```python
from build123d import *

# Parameters (mm, degrees)
F0_W     = 600
F0_H     = 600
F0_R     = 19
F1_DEPTH = 10


with BuildPart() as f1:
    # F0 (on Top) → F1 (new body)
    with BuildSketch(Plane.XY):
        with Locations((24.970765, 120.387087)):
            Rectangle(F0_W, F0_H)
        with Locations((-220.029235, -124.612913)):
            Circle(F0_R, mode=Mode.SUBTRACT)
        with Locations((-100.029235, -124.612913)):
            Circle(F0_R, mode=Mode.SUBTRACT)
        with Locations((19.970765, -124.612913)):
            Circle(F0_R, mode=Mode.SUBTRACT)
        with Locations((-220.029235, -4.612913)):
            Circle(F0_R, mode=Mode.SUBTRACT)
        with Locations((-220.029235, 115.387087)):
            Circle(F0_R, mode=Mode.SUBTRACT)
        with Locations((-100.029235, -4.612913)):
            Circle(F0_R, mode=Mode.SUBTRACT)
        with Locations((19.970765, -4.612913)):
            Circle(F0_R, mode=Mode.SUBTRACT)
        with Locations((-100.029235, 115.387087)):
            Circle(F0_R, mode=Mode.SUBTRACT)
        with Locations((19.970765, 115.387087)):
            Circle(F0_R, mode=Mode.SUBTRACT)
        with Locations((139.970765, -124.612913)):
            Circle(F0_R, mode=Mode.SUBTRACT)
        with Locations((259.970765, -124.612913)):
            Circle(F0_R, mode=Mode.SUBTRACT)
        with Locations((139.970765, -4.612913)):
            Circle(F0_R, mode=Mode.SUBTRACT)
        with Locations((139.970765, 115.387087)):
            Circle(F0_R, mode=Mode.SUBTRACT)
        with Locations((259.970765, -4.612913)):
            Circle(F0_R, mode=Mode.SUBTRACT)
        with Locations((259.970765, 115.387087)):
            Circle(F0_R, mode=Mode.SUBTRACT)
        with Locations((-220.029235, 235.387087)):
            Circle(F0_R, mode=Mode.SUBTRACT)
        with Locations((-100.029235, 235.387087)):
            Circle(F0_R, mode=Mode.SUBTRACT)
        with Locations((19.970765, 235.387087)):
            Circle(F0_R, mode=Mode.SUBTRACT)
        with Locations((-220.029235, 355.387087)):
            Circle(F0_R, mode=Mode.SUBTRACT)
        with Locations((-100.029235, 355.387087)):
            Circle(F0_R, mode=Mode.SUBTRACT)
        with Locations((19.970765, 355.387087)):
            Circle(F0_R, mode=Mode.SUBTRACT)
        with Locations((139.970765, 235.387087)):
            Circle(F0_R, mode=Mode.SUBTRACT)
        with Locations((259.970765, 235.387087)):
            Circle(F0_R, mode=Mode.SUBTRACT)
        with Locations((139.970765, 355.387087)):
            Circle(F0_R, mode=Mode.SUBTRACT)
        with Locations((259.970765, 355.387087)):
            Circle(F0_R, mode=Mode.SUBTRACT)
    extrude(amount=-F1_DEPTH)


solid = f1.part
```
Can you work these out from the model? Positions are in its coordinate system, mm. Round coordinates to 2 decimals unless told otherwise and drop trailing zeros. Order: outer loops, then holes, each group sorted by start corner. A loop starts at its lowest first (then second) coordinate and runs counter-clockwise, first axis right, second up. Notation, with made-up numbers: (63, 8.25) -> (84, 8.25) arc R9 cw to (84, 13.25) -> close; hole circle Ø10 at (55, 7). An arc over 180 degrees is marked (long way). Return JSON: item names as keys, results as strings. Group by question number.
1. If we section it at A-A, the plane y = -15.5: Write out the boundary of the cut face in (x, z).
2. If we section it at B-B, the plane z = -5.75: Count the separate pieces of the cut face and the enclosed holes in it, then the cut area to 3 significant figures.
3. Will this pin go through, and if not, where does the flat tip stop? pin 1 (23 mm diameter, centred on x = -220.03, y = -4.61, fed in from +Z).
4. I need wall thicknesses on line 1 (Y direction, x = -223, z = -6.5); line 2 (Y direction, x = 245, z = -7.75); line 3 (X direction, y = 131.5, z = -5.75). Which ranges of each line are inside material? Lowest first, please. Write a range as [from, to].
5. We'd pull the mould along Y, two halves only. Please class faces 1 (the face through (21, 191, 0)), 2 (the face through (-239.01, -3.78, -4.93)), 3 (the face through (158.093, 121.094, -4.93)): released by +Y, released by -Y, zero draft, split by the parting line, or undercut.
Output values:
{
 "1": {"outline": "(-275.03, -10) -> (-235.6, -10) -> (-235.6, 0) -> (-275.03, 0) -> close; (-204.46, -10) -> (-115.6, -10) -> (-115.6, 0) -> (-204.46, 0) -> close; (-84.46, -10) -> (4.4, -10) -> (4.4, 0) -> (-84.46, 0) -> close; (35.54, -10) -> (124.4, -10) -> (124.4, 0) -> (35.54, 0) -> close; (155.54, -10) -> (244.4, -10) -> (244.4, 0) -> (155.54, 0) -> close; (275.54, -10) -> (324.97, -10) -> (324.97, 0) -> (275.54, 0) -> close"},
 "2": {"separate pieces": "1", "enclosed holes": "25", "area": "332,000 mm²"},
 "3": {"pin 1": "through"},
 "4": {"line 1": "[-179.61, -143.38], [-105.85, -23.38], [14.15, 96.62], [134.15, 216.62], [254.15, 336.62], [374.15, 420.39]", "line 2": "[-179.61, -136.31], [-112.91, -16.31], [7.09, 103.69], [127.09, 223.69], [247.09, 343.69], [367.09, 420.39]", "line 3": "[-275.03, -230.1], [-209.96, -110.1], [-89.96, 9.9], [30.04, 129.9], [150.04, 249.9], [270.04, 324.97]"},
 "5": {"face 1": "zero draft", "face 2": "undercut", "face 3": "undercut"}
}
